```python
from build123d import *

# Parameters (mm, degrees)
BOSS_EXTRUDE1_DEPTH = 13
CUT_EXTRUDE1_DEPTH  = 73.759879054
CUT_EXTRUDE2_DEPTH  = 72.575135347
FILLET1_R           = 3
FILLET2_R           = 3


with BuildPart() as part:
    # Sketch1 → Boss-Extrude1 (new body)
    with BuildSketch(Plane.XY):
        Polygon((0, 0), (3, 0), (3, 65), (-27, 65), (-27, 62), (0, 62), align=None)
    extrude(amount=BOSS_EXTRUDE1_DEPTH)

    # Sketch6 → Cut-Extrude1 (cut, through all)
    with BuildSketch(Plane(origin=(3, 0, 0), x_dir=(0, 0, -1), z_dir=(1, 0, 0))):
        with BuildLine():
            Line((-4.95, 57.45), (-4.95, 5.05))
            ThreePointArc((-4.95, 5.05), (-6.5, 3.5), (-8.05, 5.05))
            Line((-8.05, 5.05), (-8.05, 57.45))
            ThreePointArc((-8.05, 57.45), (-6.5, 59), (-4.95, 57.45))
        make_face()
    extrude(amount=-CUT_EXTRUDE1_DEPTH, mode=Mode.SUBTRACT)

    # Sketch7 → Cut-Extrude2 (cut, through all)
    with BuildSketch(Plane(origin=(0, 65, 0), x_dir=(1, 0, 0), z_dir=(0, 1, 0))):
        with BuildLine():
            Line((-21.95, -4.95), (-4.55, -4.95))
            ThreePointArc((-4.55, -4.95), (-3, -6.5), (-4.55, -8.05))
            Line((-4.55, -8.05), (-21.95, -8.05))
            ThreePointArc((-21.95, -8.05), (-23.5, -6.5), (-21.95, -4.95))
        make_face()
    extrude(amount=-CUT_EXTRUDE2_DEPTH, mode=Mode.SUBTRACT)

    # Fillet1
    fillet1_edges = [part.edges().sort_by_distance(p)[0] for p in [
        (0, 62, 6.5),
    ]]
    fillet(fillet1_edges, radius=FILLET1_R - 0.0001)  # a hair under: the kernel refuses the full size

    # Fillet2
    fillet2_edges = [part.edges().sort_by_distance(p)[0] for p in [
        (-27, 63.5, 13),
        (-27, 63.5, 0),
        (1.5, 0, 0),
        (1.5, 0, 13),
    ]]
    fillet(fillet2_edges, radius=FILLET2_R)


solid = part.part
```
Can you work these out from the model? Positions are in its coordinate system, mm. A direction names the side the tool comes from. Coordinates: 2 decimals unless noted, no trailing zeros. Loops run counter-clockwise (first coordinate to the right, second up) from the corner with the lowest first, then second, coordinate; pieces in that order, holes last.
1) I need wall thicknesses on probe 1 along Z at (x, y) = (0.25, 28); probe 2 along Y at (x, z) = (-2.75, 5.75). Which ranges of each line are inside material? Lowest first, please.
2) Imagine slicing it at C-C on x = -12.5. List the corners of the cut face in (y, z) for me, plus the area to 3 significant figures.
3) Thinking about a two-plate mould opening in Z: for faces 1 (the cylindrical face through (-26.1, 63.48, 12.14)), 2 (the flat face through (1, 0, 6)), 3 (the cylindrical face through (-3, 63.5, 6.5)), which applies, pulls with the +Z half, pulls with the -Z half, needs draft (parallel to the pull), parting line crosses it, or undercut?
4) Imagine slicing it at B-B on z = 6.5. State how many separate pieces and enclosed holes the cut face has, plus the area to 3 significant figures.
5) For pin 1 (4 mm diameter, centred on y = 38, z = 4, fed in from -X); pin 2 (6.5 mm diameter, centred on x = -12.5, z = 7, fed in from -Y), each with a flat end and sliding along its axis, tell me the tip position at first contact or that it passes through.
6) Imagine slicing it at A-A on y = 27. List the corners of the cut face in (x, z) for me.
7) Which directions (+Z, -Z, +X, -X, +Y, -Y) give clear straight access to the entire face, cutting with the end or side of a thin tool? Please do faces 4 (the flat face through (-13, 64, 8.05)), 5 (the flat face through (0, 30, 4)), 6 (the flat face through (2, 32, 4.95)).
Completed:
1. probe 1: z = 0 to 4.95, 8.05 to 13
1. probe 2: y = 61.99 to 65
2. outline: (62, 0) - (65, 0) - (65, 4.95) - (62, 4.95) - close; (62, 8.05) - (65, 8.05) - (65, 13) - (62, 13) - close
2. area: 29.7 mm2
3. face 1: pulls with the +Z half
3. face 2: needs draft
3. face 3: undercut
4. separate pieces: 3
4. enclosed holes: 0
4. area: 49.9 mm2
5. pin 1: stops at x = 0
5. pin 2: stops at y = 62
6. outline: (0, 0) - (3, 0) - (3, 4.95) - (0, 4.95) - close; (0, 8.05) - (3, 8.05) - (3, 13) - (0, 13) - close
7. face 4: +Y, -Y
7. face 5: +Z, -Z, -X, -Y
7. face 6: +X, -X
